Build history of the part. All positions in model axes, mm. Face numbers are marked on the shaded views. A direction names the side the tool comes from. Coordinates: 2 decimals unless noted, no trailing zeros. Order: outer loops, then holes, each group sorted by start corner. A loop starts at its lowest first (then second) coordinate and runs counter-clockwise, first axis right, second up. Notation, with made-up numbers: (40, 86) -> (65, 86) arc R8 ccw to (65, 98) -> close; hole circle Ø6 at (68, 67). An arc over 180 degrees is marked (long way). Write each question's results on one line, items separated by ' | '.
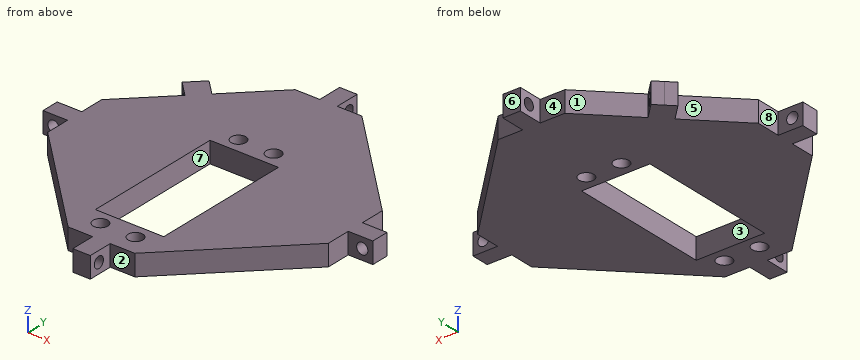
from build123d import *

# Parameters (mm, degrees)
SKETCH_1_R          = 2.1
SKETCH_1_W          = 5
SKETCH_1_H          = 7
SKETCH_1_W_2        = 7
SKETCH_1_H_2        = 5
SKETCH_1_W_3        = 19.5
SKETCH_1_H_3        = 6.75
EXTRUDE_2_DEPTH     = 6
SKETCH_2_R          = 1.6
CUT_EXTRUDE_1_DEPTH = 5
SKETCH_3_R          = 1.6
CUT_EXTRUDE_2_DEPTH = 5
SKETCH_4_R          = 1.6
CUT_EXTRUDE_3_DEPTH = 5
SKETCH_5_R          = 1.6
CUT_EXTRUDE_4_DEPTH = 5
EXTRUDE_3_DEPTH     = 6
SKETCH_7_R          = 1.6
CUT_EXTRUDE_5_DEPTH = 6


with BuildPart() as part:
    # 草图1 → 凸台-拉伸2 (new body)
    # profile 1 of 6: a face of its own
    with BuildSketch(Plane.XY):
        Polygon((-9.5, 39.997474683), (-39.997474683, 9.5), (-39.997474683, 2.5), (-39.997474683, -2.5), (-39.997474683, -9.5), (-9.5, -39.997474683), (-2.5, -39.997474683), (2.5, -39.997474683), (9.5, -39.997474683), (39.997474683, -9.5), (39.997474683, -2.5), (39.997474683, 2.5), (39.997474683, 9.5), (9.5, 39.997474683), (2.5, 39.997474683), (-2.5, 39.997474683), align=None)
        Polygon((-9.75, -30.1), (-9.75, 10.3), (9.75, 10.3), (9.75, -30.1), (9.75, -36.85), (-9.75, -36.85), align=None, mode=Mode.SUBTRACT)
        with Locations((-5, 14.465)):
            Circle(SKETCH_1_R, mode=Mode.SUBTRACT)
        with Locations((5, 14.465)):
            Circle(SKETCH_1_R, mode=Mode.SUBTRACT)
    # profile 2 of 6: a face of its own
    with BuildSketch(Plane.XY):
        with Locations((0, 43.497474683)):
            Rectangle(SKETCH_1_W, SKETCH_1_H)
    # profile 3 of 6: a face of its own
    with BuildSketch(Plane.XY):
        with Locations((-43.497474683, 0)):
            Rectangle(SKETCH_1_W_2, SKETCH_1_H_2)
    # profile 4 of 6: a face of its own
    with BuildSketch(Plane.XY):
        with Locations((0, -43.497474683)):
            Rectangle(SKETCH_1_W, SKETCH_1_H)
    # profile 5 of 6: a face of its own
    with BuildSketch(Plane.XY):
        with Locations((43.497474683, 0)):
            Rectangle(SKETCH_1_W_2, SKETCH_1_H_2)
    # profile 6 of 6: a face of its own
    with BuildSketch(Plane.XY):
        with Locations((0, -33.475)):
            Rectangle(SKETCH_1_W_3, SKETCH_1_H_3)
        with Locations((5, -34.165)):
            Circle(SKETCH_1_R, mode=Mode.SUBTRACT)
        with Locations((-5, -34.165)):
            Circle(SKETCH_1_R, mode=Mode.SUBTRACT)
    extrude(amount=EXTRUDE_2_DEPTH)

    # 草图2 → 切除-拉伸1 (cut)
    with BuildSketch(Plane.XZ.offset(2.5)):
        with Locations((-43.997474683, 3)):
            Circle(SKETCH_2_R)
    extrude(amount=-CUT_EXTRUDE_1_DEPTH, mode=Mode.SUBTRACT)

    # 草图3 → 切除-拉伸2 (cut)
    with BuildSketch(Plane(origin=(2.5, 0, 0), x_dir=(0, 0, -1), z_dir=(1, 0, 0))):
        with Locations(Location((-3, -43.997474683, 0), (0, 0, 90))):
            Circle(SKETCH_3_R)
    extrude(amount=-CUT_EXTRUDE_2_DEPTH, mode=Mode.SUBTRACT)

    # 草图4 → 切除-拉伸3 (cut)
    with BuildSketch(Plane(origin=(0, 2.5, 0), x_dir=(1, 0, 0), z_dir=(0, 1, 0))):
        with Locations(Location((43.997474683, -3, 0), (0, 0, 180))):
            Circle(SKETCH_4_R)
    extrude(amount=-CUT_EXTRUDE_3_DEPTH, mode=Mode.SUBTRACT)

    # 草图5 → 切除-拉伸4 (cut)
    with BuildSketch(Plane.ZY.offset(2.5)):
        with Locations(Location((3, 43.997474683, 0), (0, 0, 270))):
            Circle(SKETCH_5_R)
    extrude(amount=-CUT_EXTRUDE_4_DEPTH, mode=Mode.SUBTRACT)

    # 草图6 → 凸台-拉伸3 (add)
    with BuildSketch(Plane.XY.offset(6)):
        Polygon((-26.870057685, 22.627416998), (-24.748737342, 24.748737342), (-28.991378029, 28.991378029), (-31.112698372, 26.870057685), align=None)
        Polygon((-24.748737342, 24.748737342), (-22.627416998, 26.870057685), (-26.870057685, 31.112698372), (-28.991378029, 28.991378029), align=None)
    extrude(amount=-EXTRUDE_3_DEPTH)

    # 草图7 → 切除-拉伸5 (cut)
    with BuildSketch(Plane(origin=(-2.121320344, -2.121320344, 0), x_dir=(0, 0, 1), z_dir=(-0.7071067811865471, -0.7071067811865479, 0))):
        with Locations(Location((3, 38, 0), (0, 0, 270))):
            Circle(SKETCH_7_R)
    extrude(amount=-CUT_EXTRUDE_5_DEPTH, mode=Mode.SUBTRACT)


solid = part.part
Item 1: Pull direction X, two halves, no side cores. Call the marked faces 6, 7 and 8: released by +X, released by -X, zero draft, split by the parting line, or undercut.
Answer:
face 6: zero draft | face 7: undercut | face 8: released by -X
Item 2: Drill centre lines: line 1 (Y direction, x = 5, z = 2.5) (3 decimals); line 2 (Y direction, x = 2, z = 1.8); line 3 (X direction, y = -33, z = 2.8). Where is each one in solid material? Low to high. Write a range as from..to.
Answer:
line 1: y = -39.997..-36.265, -32.065..-30.1, 10.3..12.365, 16.565..39.997 | line 2: y = -47..-45.06, -42.94..-30.1, 10.3..42.94, 45.06..47 | line 3: x = -16.5..-6.75, -3.25..3.25, 6.75..16.5
Item 3: Pin check, flat tips, straight feed: pin 1 (1.8 mm diameter, centred on x = -5.5, z = 4, fed in from -Y); pin 2 (3 mm diameter, centred on x = -6, z = 2.5, fed in from +Y); pin 3 (3 mm diameter, centred on x = -44, z = 4.5, fed in from -Y); pin 4 (5 mm diameter, centred on x = -5, y = -34.165, fed in from +Z). Stop position of each tip, or through.
Answer:
pin 1: stops at y = -40 | pin 2: stops at y = 40 | pin 3: stops at y = -2.5 | pin 4: stops at z = 6
Item 4: Slice it at B-B, the plane y = -14. List the corners of the cut face in (x, z).
Answer:
outline: (-35.5, 0) -> (-9.75, 0) -> (-9.75, 6) -> (-35.5, 6) -> close; (9.75, 0) -> (35.5, 0) -> (35.5, 6) -> (9.75, 6) -> close
Item 5: Slice it at C-C, the plane z = 3. State how many separate pieces and enclosed holes the cut face has, and give its area (3 significant figures).
Answer:
separate pieces: 6 | enclosed holes: 5 | area: 3,790 mm^2
Item 6: Slice it at A-A, the plane x = -5. List the corners of the cut face in (y, z) (3 decimals).
Answer:
outline: (-39.997, 0) -> (-36.265, 0) -> (-36.265, 6) -> (-39.997, 6) -> close; (-32.065, 0) -> (-30.1, 0) -> (-30.1, 6) -> (-32.065, 6) -> close; (10.3, 0) -> (12.365, 0) -> (12.365, 6) -> (10.3, 6) -> close; (16.565, 0) -> (39.997, 0) -> (39.997, 6) -> (16.565, 6) -> close
Item 7: Tool access for the marked faces 1, 2, 3, 4 and 5: list every direction of +Z, -Z, +X, -X, +Y, -Y with a clear straight run to the whole face (end or side of a thin tool).
Answer:
face 1: +Z, -Z, +Y | face 2: +Z, -Z, +X, -Y | face 3: +Z, -Z | face 4: +Z, -Z, -X, +Y | face 5: +Z, -Z, -X
Item 8: Slice it at D-D, the plane y = 18. List the corners of the cut face in (x, z), and give its area (3 significant figures).
Answer:
outline: (-31.5, 0) -> (31.5, 0) -> (31.5, 6) -> (-31.5, 6) -> close | area: 378 mm^2
